Geometry: see drawing. Coordinates: mm, zero at the bounding-box minimum. Give positions to 0.01 mm unless a question says otherwise; leave off trailing zeros. Loops run counter-clockwise (first coordinate to the right, second up) from the corner with the lowest first, then second, coordinate; pieces in that order, holes last. Notation, with made-up numbers: (78.25, 61.5) -> (93.25, 61.5) arc R8 ccw to (93.25, 69.5) -> close; hole circle Ø7 at (53.25, 32.5). An arc over 180 degrees is marked (long way). Answer in a Markdown table with one row per item. Add a question column.
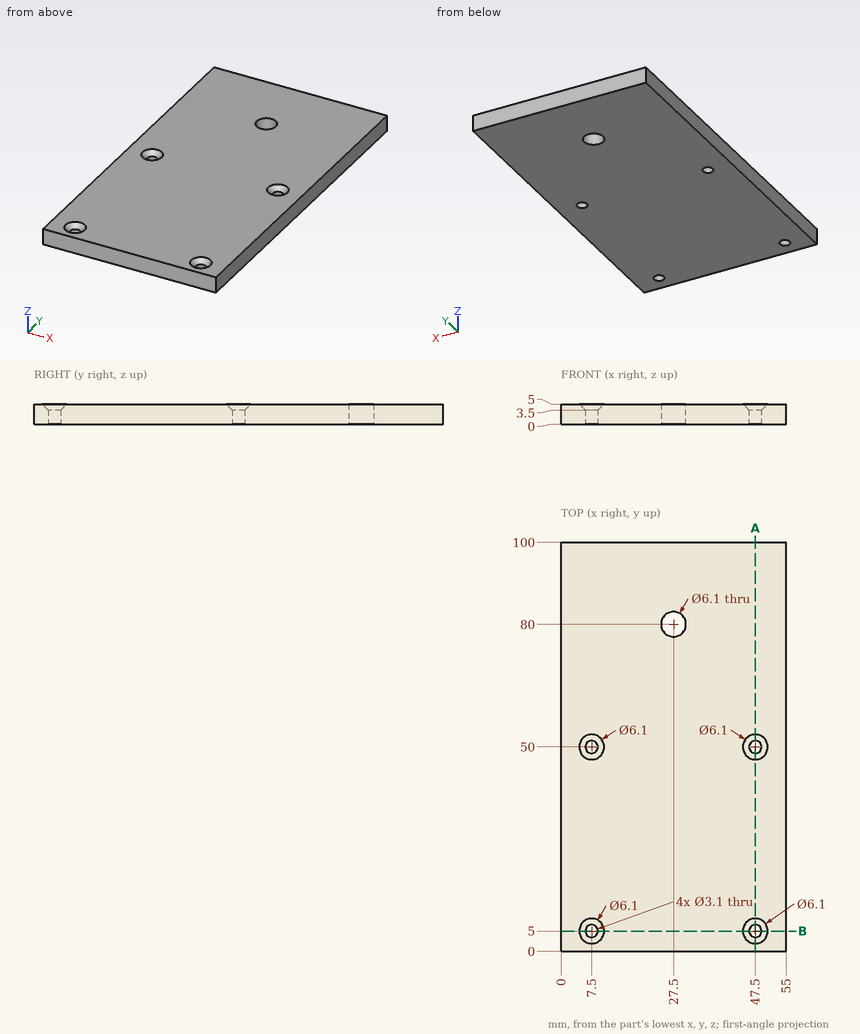
1) Section B-B on y = 5. Output: boundary loops of the cut face in (x, z).
2) Pin query (flat end, axial travel): pin 1 (3 mm diameter, centred on x = 47.5, y = 50, fed in from +Z) (1 decimal). Return the tip coordinate at first contact, or that it passes through.
3) Section A-A on x = 47.5. Output: boundary loops of the cut face in (y, z), and give its area (4 significant figures).
4) Material intervals for line 1 along Y through (x, z) = (7.5, 2.1), sorted ascending.
Working result:
| question | item | result |
|---|---|---|
| 1 | outline | (0, 0) -> (5.95, 0) -> (5.95, 3.5) -> (4.45, 5) -> (0, 5) -> close; (9.05, 0) -> (45.95, 0) -> (45.95, 3.5) -> (44.45, 5) -> (10.55, 5) -> (9.05, 3.5) -> close; (49.05, 0) -> (55, 0) -> (55, 5) -> (50.55, 5) -> (49.05, 3.5) -> close |
| 2 | pin 1 | passes through |
| 3 | outline | (0, 0) -> (3.45, 0) -> (3.45, 3.5) -> (1.95, 5) -> (0, 5) -> close; (6.55, 0) -> (48.45, 0) -> (48.45, 3.5) -> (46.95, 5) -> (8.05, 5) -> (6.55, 3.5) -> close; (51.55, 0) -> (100, 0) -> (100, 5) -> (53.05, 5) -> (51.55, 3.5) -> close |
| 3 | area | 464.5 mm2 |
| 4 | line 1 | y = 0 to 3.45, 6.55 to 48.45, 51.55 to 100 |
